from build123d import *

# Parameters (mm, degrees)
SKETCH1_R           = 14.351
SKETCH1_R_2         = 2.413
BOSS_EXTRUDE1_DEPTH = 3.175


with BuildPart() as part:
    # Sketch1 → Boss-Extrude1 (new body)
    with BuildSketch(Plane.XY):
        with BuildLine():
            Line((-31.75, 34.29), (31.75, 34.29))
            ThreePointArc((31.75, 34.29), (66.04, 0), (31.75, -34.29))
            Line((31.75, -34.29), (-31.75, -34.29))
            ThreePointArc((-31.75, -34.29), (-66.04, 0), (-31.75, 34.29))
        make_face()
        with Locations((-31.75, 0)):
            Circle(SKETCH1_R, mode=Mode.SUBTRACT)
        with Locations(Location((31.75, 0, 0), (0, 0, 180))):
            Circle(SKETCH1_R, mode=Mode.SUBTRACT)
        with Locations((-19.506383886, 14.177461716)):
            Circle(SKETCH1_R_2, mode=Mode.SUBTRACT)
        with Locations(Location((19.506383886, 14.177461716, 0), (0, 0, 180))):
            Circle(SKETCH1_R_2, mode=Mode.SUBTRACT)
    extrude(amount=BOSS_EXTRUDE1_DEPTH)


solid = part.part
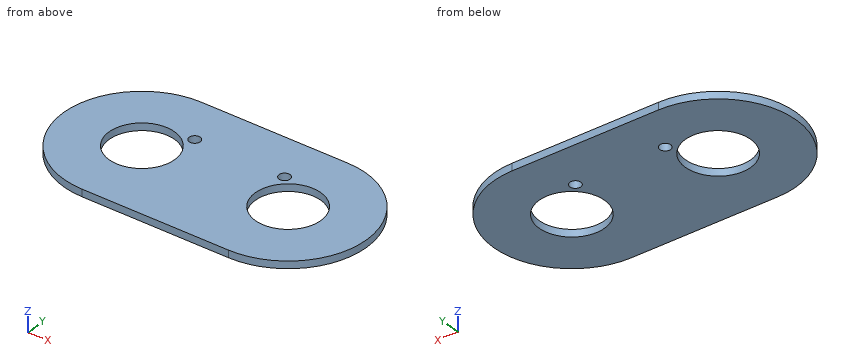
Work out the finished part from the listing and answer in its coordinate system (mm). Round coordinates to 2 decimals unless told otherwise and drop trailing zeros. Write each loop counter-clockwise with the first axis right and the second up, starting at its lowest first coordinate (ties: lowest second). Pieces come first, ordered by that corner, then holes. Notation, with made-up numbers: M 30,-32.5 L 58,-32.5 A27 ccw 58,1.5 Z; hole C 67.25,14.25 d7. An arc over 180 degrees is marked long. Use a Markdown table: item, result.
1) The part is cut by section D-D on x = 51. Give the vertices of the cut face in (y, z) (3 decimals).
Taken from the geometry:
| item | result |
|---|---|
| outline | M -28.377,0 L 28.377,0 L 28.377,3.175 L -28.377,3.175 Z |
2) The part is cut by section B-B on x = -37. Give the vertices of the cut face in (y, z) (3 decimals).
Taken from the geometry:
| item | result |
|---|---|
| outline | M -33.886,0 L -13.356,0 L -13.356,3.175 L -33.886,3.175 Z; M 13.356,0 L 33.886,0 L 33.886,3.175 L 13.356,3.175 Z |
3) Consider line 1 (X direction, y = 12, z = 1.55); line 2 (X direction, y = 10, z = 1.6); line 3 (X direction, y = -9, z = 0.3). Determine where each line is inside the solid, lowest interval first. Write a range as [from, to].
Taken from the geometry:
| item | result |
|---|---|
| line 1 | x = [-63.87, -39.62], [-23.88, -20.55], [-18.47, 18.47], [20.55, 23.88], [39.62, 63.87] |
| line 2 | x = [-64.55, -42.04], [-21.46, 21.46], [42.04, 64.55] |
| line 3 | x = [-64.84, -42.93], [-20.57, 20.57], [42.93, 64.84] |
4) The part is cut by section C-C on z = 2.5. Give the vertices of the cut face in (x, y).
Taken from the geometry:
| item | result |
|---|---|
| outline | M -31.75,-34.29 L 31.75,-34.29 A34.29 ccw 31.75,34.29 L -31.75,34.29 A34.29 ccw Z; hole C -31.75,0 d28.7; hole C -19.51,14.18 d4.83; hole C 19.51,14.18 d4.83; hole C 31.75,0 d28.7 |
5) Flat-ended cylindrical pins translate along their axes: pin 1 (1 mm diameter, centred on y = 14, z = 2, fed in from +X); pin 2 (17 mm diameter, centred on x = 31.75, y = 0, fed in from -Z). Find the tip coordinate at first contact, or state that the pin passes through.
Taken from the geometry:
| item | result |
|---|---|
| pin 1 | stops at x = 63.27 |
| pin 2 | passes through |
6) The part is cut by section A-A on y = 0. Give the vertices of the cut face in (x, z) (3 decimals), plus the area to 3 significant figures.
Taken from the geometry:
| item | result |
|---|---|
| outline | M -66.04,0 L -46.101,0 L -46.101,3.175 L -66.04,3.175 Z; M -17.399,0 L 17.399,0 L 17.399,3.175 L -17.399,3.175 Z; M 46.101,0 L 66.04,0 L 66.04,3.175 L 46.101,3.175 Z |
| area | 237 mm2 |
